from build123d import *

# Parameters (mm, degrees)
SKETCH_1_R          = 1.65
SKETCH_1_R_2        = 6.85
EXTRUDE_1_DEPTH     = 3
FILLET_1_R          = 10
SKETCH_2_W          = 40
SKETCH_2_H          = 72.562953015
CUT_EXTRUDE_1_DEPTH = 10


with BuildPart() as part:
    # 草图1 → 凸台-拉伸1 (new body)
    with BuildSketch(Plane(origin=(0, 0, 0), x_dir=(1, 0, 0), z_dir=(0, 1, 0))):
        Polygon((0, 0), (0, 50.01), (40, 50.01), (40, 0), (40, -89.81), (0, -89.81), align=None)
        with Locations(Location((20, -1.7, 0), (0, 0, 270))):
            Circle(SKETCH_1_R, mode=Mode.SUBTRACT)
        with Locations(Location((20, -38.1, 0), (0, 0, 270))):
            Circle(SKETCH_1_R, mode=Mode.SUBTRACT)
        with Locations(Location((20, 31.62, 0), (0, 0, 270))):
            Circle(SKETCH_1_R, mode=Mode.SUBTRACT)
        with Locations(Location((27.794228634, 18.12, 0), (0, 0, 270))):
            Circle(SKETCH_1_R, mode=Mode.SUBTRACT)
        with Locations(Location((12.205771366, 18.12, 0), (0, 0, 270))):
            Circle(SKETCH_1_R, mode=Mode.SUBTRACT)
        with Locations(Location((27.794228634, -57.92, 0), (0, 0, 270))):
            Circle(SKETCH_1_R, mode=Mode.SUBTRACT)
        with Locations(Location((12.205771366, -57.92, 0), (0, 0, 270))):
            Circle(SKETCH_1_R, mode=Mode.SUBTRACT)
        with Locations(Location((20, -71.42, 0), (0, 0, 270))):
            Circle(SKETCH_1_R, mode=Mode.SUBTRACT)
        with Locations(Location((20, 22.62, 0), (0, 0, 270))):
            Circle(SKETCH_1_R_2, mode=Mode.SUBTRACT)
        with Locations(Location((20, -62.42, 0), (0, 0, 270))):
            Circle(SKETCH_1_R_2, mode=Mode.SUBTRACT)
        with BuildLine():
            Line((5, 0), (13, 0))
            ThreePointArc((13, 0), (14.7, -1.7), (13, -3.4))
            Line((13, -3.4), (5, -3.4))
            ThreePointArc((5, -3.4), (3.3, -1.7), (5, 0))
        make_face(mode=Mode.SUBTRACT)
        with BuildLine():
            Line((27, 0), (35, 0))
            ThreePointArc((35, 0), (36.7, -1.7), (35, -3.4))
            Line((35, -3.4), (27, -3.4))
            ThreePointArc((27, -3.4), (25.3, -1.7), (27, 0))
        make_face(mode=Mode.SUBTRACT)
        with BuildLine():
            Line((27, -39.8), (35, -39.8))
            ThreePointArc((35, -39.8), (36.7, -38.1), (35, -36.4))
            Line((35, -36.4), (27, -36.4))
            ThreePointArc((27, -36.4), (25.3, -38.1), (27, -39.8))
        make_face(mode=Mode.SUBTRACT)
        with BuildLine():
            Line((5, -39.8), (13, -39.8))
            ThreePointArc((13, -39.8), (14.7, -38.1), (13, -36.4))
            Line((13, -36.4), (5, -36.4))
            ThreePointArc((5, -36.4), (3.3, -38.1), (5, -39.8))
        make_face(mode=Mode.SUBTRACT)
    extrude(amount=EXTRUDE_1_DEPTH)

    # 圆角1
    fillet_1_edges = [part.edges().sort_by_distance(p)[0] for p in [
        (0, 1.5, -50.01),
        (40, 1.5, -50.01),
        (40, 1.5, 89.81),
        (0, 1.5, 89.81),
    ]]
    fillet(fillet_1_edges, radius=FILLET_1_R)

    # 草图2 → 切除-拉伸1 (cut)
    with BuildSketch(Plane(origin=(0, 3, 0), x_dir=(1, 0, 0), z_dir=(0, 1, 0))):
        with Locations((20, 41.281476508)):
            Rectangle(SKETCH_2_W, SKETCH_2_H)
    extrude(amount=-CUT_EXTRUDE_1_DEPTH, mode=Mode.SUBTRACT)


solid = part.part
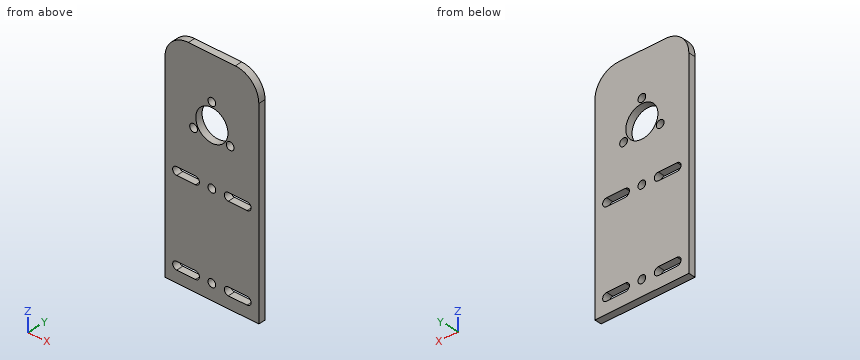
Can you work these out from the model? Positions are in its coordinate system, mm. Coordinates: 2 decimals unless noted, no trailing zeros. Write each loop counter-clockwise with the first axis right and the second up, starting at its lowest first coordinate (ties: lowest second). Pieces come first, ordered by that corner, then holes. Notation, with made-up numbers: (47.25, 2.5) - (77.25, 2.5) arc R21 ccw to (77.25, 27.5) - close; hole circle Ø1 at (-36.75, 85). An arc over 180 degrees is marked (long way). Return JSON: item names as keys, results as strings. Group by question number.
Item 1: If we section it at C-C (x = 20): Write out the boundary of the cut face in (y, z).
Item 2: If we section it at A-A (z = 71.42): Write out the boundary of the cut face in (x, y).
Item 3: If we section it at D-D (x = 6): Write out the boundary of the cut face in (y, z), then the cut area to 3 significant figures.
Item 4: Please list where these lines run through material, in increasing order: probe 1 along Z at (x, y) = (10.5, 0.2); probe 2 along X at (y, z) = (1.9, 57.92); probe 3 along Z at (x, y) = (36.5, 0.4).
Item 5: I'm going to push flat-ended pins straight in: pin 1 Ø5.5 at (x, z) = (12.21, 57.92) entering from +Y; pin 2 Ø2.5 at (x, z) = (20, 1.7) entering from -Y. Where does each tip first touch, or does it pass through?
Item 6: If we section it at B-B (z = 1.7): Write out the boundary of the cut face in (x, y), then the cut area to 3 significant figures.
Return value:
{
 "1": {"outline": "(0, -5) - (3, -5) - (3, 0.05) - (0, 0.05) - close; (0, 3.35) - (3, 3.35) - (3, 36.45) - (0, 36.45) - close; (0, 39.75) - (3, 39.75) - (3, 55.57) - (0, 55.57) - close; (0, 69.27) - (3, 69.27) - (3, 69.77) - (0, 69.77) - close; (0, 73.07) - (3, 73.07) - (3, 89.81) - (0, 89.81) - close"},
 "2": {"outline": "(0, 0) - (18.35, 0) - (18.35, 3) - (0, 3) - close; (21.65, 0) - (40, 0) - (40, 3) - (21.65, 3) - close"},
 "3": {"outline": "(0, -5) - (3, -5) - (3, 0) - (0, 0) - close; (0, 3.4) - (3, 3.4) - (3, 36.4) - (0, 36.4) - close; (0, 39.8) - (3, 39.8) - (3, 88.98) - (0, 88.98) - close", "area": "262 mm^2"},
 "4": {"probe 1": "z = -5 to 0, 3.4 to 36.4, 39.8 to 89.81", "probe 2": "x = 0 to 10.56, 13.86 to 14.84, 25.16 to 26.14, 29.44 to 40", "probe 3": "z = -5 to 0.9, 2.5 to 37.3, 38.9 to 87.41"},
 "5": {"pin 1": "stops at y = 3", "pin 2": "passes through"},
 "6": {"outline": "(0, 0) - (3.3, 0) - (3.3, 3) - (0, 3) - close; (14.7, 0) - (18.35, 0) - (18.35, 3) - (14.7, 3) - close; (21.65, 0) - (25.3, 0) - (25.3, 3) - (21.65, 3) - close; (36.7, 0) - (40, 0) - (40, 3) - (36.7, 3) - close", "area": "41.7 mm^2"}
}
